```python
from build123d import *

# Parameters (mm, degrees)
BOSS_EXTRU_1_DEPTH      = 6
CONG_1_R                = 3
CONG_2_R                = 20
ENL_V_MAT_EXTRU_1_REACH = 118.402
ESQUISSE2_R             = 1.45
ENL_V_MAT_EXTRU_2_REACH = 118.402
CONG_3_R                = 1.5
ESQUISSE4_R             = 1.45
ENL_V_MAT_EXTRU_3_DEPTH = 6
ESQUISSE5_R             = 1.15
ENL_V_MAT_EXTRU_4_DEPTH = 6


with BuildPart() as part:
    # Esquisse1 → Boss.-Extru.1 (new body)
    with BuildSketch(Plane.XY):
        with BuildLine():
            Line((-14, -30), (-5.970001079, -110))
            ThreePointArc((-5.970001079, -110), (0, -115.400761222), (5.970001079, -110))
            Line((5.970001079, -110), (14, -30))
            Line((14, -30), (14, -18))
            Line((14, -18), (-6, -18))
            Line((-6, -18), (-6, 22))
            Line((-6, 22), (14, 22))
            Line((14, 22), (14, 30))
            Line((14, 30), (-14, 30))
            Line((-14, 30), (-14, -30))
        make_face()
    extrude(amount=BOSS_EXTRU_1_DEPTH)

    # Congé1
    cong_1_edges = [part.edges().sort_by_distance(p)[0] for p in [
        (-14, 30, 3),
        (14, 30, 3),
    ]]
    fillet(cong_1_edges, radius=CONG_1_R)

    # Congé2
    cong_2_edges = [part.edges().sort_by_distance(p)[0] for p in [
        (14, -30, 3),
        (-14, -30, 3),
    ]]
    fillet(cong_2_edges, radius=CONG_2_R)

    # Esquisse2 → Enlèv. mat.-Extru.1 (cut, up to next)
    with BuildSketch(Plane.XY.offset(6), mode=Mode.PRIVATE) as enl_v_mat_extru_1_sk1:
        with Locations((9.08, -21.75)):
            Circle(ESQUISSE2_R)
    enl_v_mat_extru_1_tool1 = extrude(enl_v_mat_extru_1_sk1.sketch, amount=-ENL_V_MAT_EXTRU_1_REACH, mode=Mode.PRIVATE) & part.part
    # Esquisse2 → Enlèv. mat.-Extru.1 (cut, up to next)
    with BuildSketch(Plane.XY.offset(6), mode=Mode.PRIVATE) as enl_v_mat_extru_1_sk2:
        with Locations((-1.08, -21.75)):
            Circle(ESQUISSE2_R)
    enl_v_mat_extru_1_tool2 = extrude(enl_v_mat_extru_1_sk2.sketch, amount=-ENL_V_MAT_EXTRU_1_REACH, mode=Mode.PRIVATE) & part.part
    # Esquisse2 → Enlèv. mat.-Extru.1 (cut, up to next)
    with BuildSketch(Plane.XY.offset(6), mode=Mode.PRIVATE) as enl_v_mat_extru_1_sk3:
        with Locations((-1.08, 25.75)):
            Circle(ESQUISSE2_R)
    enl_v_mat_extru_1_tool3 = extrude(enl_v_mat_extru_1_sk3.sketch, amount=-ENL_V_MAT_EXTRU_1_REACH, mode=Mode.PRIVATE) & part.part
    # Esquisse2 → Enlèv. mat.-Extru.1 (cut, up to next)
    with BuildSketch(Plane.XY.offset(6), mode=Mode.PRIVATE) as enl_v_mat_extru_1_sk4:
        with Locations((9.08, 25.75)):
            Circle(ESQUISSE2_R)
    enl_v_mat_extru_1_tool4 = extrude(enl_v_mat_extru_1_sk4.sketch, amount=-ENL_V_MAT_EXTRU_1_REACH, mode=Mode.PRIVATE) & part.part
    add(enl_v_mat_extru_1_tool1.solids().sort_by_distance((9.08, -21.75, 6))[0], mode=Mode.SUBTRACT)
    add(enl_v_mat_extru_1_tool2.solids().sort_by_distance((-1.08, -21.75, 6))[0], mode=Mode.SUBTRACT)
    add(enl_v_mat_extru_1_tool3.solids().sort_by_distance((-1.08, 25.75, 6))[0], mode=Mode.SUBTRACT)
    add(enl_v_mat_extru_1_tool4.solids().sort_by_distance((9.08, 25.75, 6))[0], mode=Mode.SUBTRACT)

    # Esquisse3 → Enlèv. mat.-Extru.2 (cut, up to next)
    with BuildSketch(Plane.XY.offset(6), mode=Mode.PRIVATE) as enl_v_mat_extru_2_sk1:
        Polygon((-7.886583597, -31.017533633), (-4.584381628, -63.916187805), (6.894740823, -42.63737417), align=None)
    enl_v_mat_extru_2_tool1 = extrude(enl_v_mat_extru_2_sk1.sketch, amount=-ENL_V_MAT_EXTRU_2_REACH, mode=Mode.PRIVATE) & part.part
    # Esquisse3 → Enlèv. mat.-Extru.2 (cut, up to next)
    with BuildSketch(Plane.XY.offset(6), mode=Mode.PRIVATE) as enl_v_mat_extru_2_sk2:
        Polygon((6.894740823, -52.121802831), (-3.854189345, -70.511493223), (3.66385974, -84.30991259), align=None)
    enl_v_mat_extru_2_tool2 = extrude(enl_v_mat_extru_2_sk2.sketch, amount=-ENL_V_MAT_EXTRU_2_REACH, mode=Mode.PRIVATE) & part.part
    # Esquisse3 → Enlèv. mat.-Extru.2 (cut, up to next)
    with BuildSketch(Plane.XY.offset(6), mode=Mode.PRIVATE) as enl_v_mat_extru_2_sk3:
        Polygon((-2.728137467, -80.682315655), (-0.663223344, -101.254314661), (3.006387716, -91.078168987), align=None)
    enl_v_mat_extru_2_tool3 = extrude(enl_v_mat_extru_2_sk3.sketch, amount=-ENL_V_MAT_EXTRU_2_REACH, mode=Mode.PRIVATE) & part.part
    add(enl_v_mat_extru_2_tool1.solids().sort_by_distance((-1.858741, -45.857032, 6))[0], mode=Mode.SUBTRACT)
    add(enl_v_mat_extru_2_tool2.solids().sort_by_distance((2.234804, -68.98107, 6))[0], mode=Mode.SUBTRACT)
    add(enl_v_mat_extru_2_tool3.solids().sort_by_distance((-0.128324, -91.004933, 6))[0], mode=Mode.SUBTRACT)

    # Congé3
    cong_3_edges = [part.edges().sort_by_distance(p)[0] for p in [
        (6.894740823, -52.121802831, 3),
        (3.66385974, -84.30991259, 3),
        (-3.854189345, -70.511493223, 3),
        (-2.728137467, -80.682315655, 3),
        (3.006387716, -91.078168987, 3),
        (-0.663223344, -101.254314661, 3),
        (-7.886583597, -31.017533633, 3),
        (6.894740823, -42.63737417, 3),
        (-4.584381628, -63.916187805, 3),
    ]]
    fillet(cong_3_edges, radius=CONG_3_R)

    # Esquisse4 → Enlèv. mat.-Extru.3 (cut)
    with BuildSketch(Plane.XY.offset(6)):
        with Locations((0, -104.400761222)):
            Circle(ESQUISSE4_R)
    extrude(amount=-ENL_V_MAT_EXTRU_3_DEPTH, mode=Mode.SUBTRACT)

    # Esquisse5 → Enlèv. mat.-Extru.4 (cut)
    with BuildSketch(Plane.XY.offset(6)):
        with Locations((-8.41, 17)):
            Circle(ESQUISSE5_R)
        with Locations((-8.41, 7)):
            Circle(ESQUISSE5_R)
    extrude(amount=-ENL_V_MAT_EXTRU_4_DEPTH, mode=Mode.SUBTRACT)


solid = part.part
```
Input: part model. Units: mm. Frame: model coordinates. A direction names the side the tool comes from. Coordinates: 2 decimals unless noted, no trailing zeros. Loops run counter-clockwise (first coordinate to the right, second up) from the corner with the lowest first, then second, coordinate; pieces in that order, holes last. Notation, with made-up numbers: M 17,15 L 67,15 A17 ccw 67,46 Z; hole C 71.25,76.5 d7. An arc over 180 degrees is marked long. Use a Markdown table: item, result. Add a question column.
1) Set-up query: faces 5 (the cylindrical face through (-13.1, 29.14, 3.04)), 6 (the flat face through (4, 22, 3)), 7 (the flat face through (0.044, -63.842, 3.042)). Return all of +Z, -Z, +X, -X, +Y, -Y with unobstructed straight access to the full face (end or side cutting, diameter ignored); none if empty.
2) Section D-D, the plane z = 1.25. Give the number of separate pieces and of enclosed holes in the cut face, plus the area to 3 significant figures.
3) Section B-B, the plane x = 9.08. Return the cut outline in (y, z).
4) Section C-C, the plane y = -63. Return the cut outline in (x, z).
5) Line query: L1, parallel to Y at x = 0.75, z = 1.75; L2, parallel to X at y = 18, z = 4.25; L3, parallel to X at y = -73.5, z = 5. Output: solid intervals per line, ascending. Write a range as from..to.
6) Draft query along X for faces 1 (the cylindrical face through (-0.1, -115.4, 3)), 2 (the cylindrical face through (5.21, -57.41, 2.96)), 3 (the cylindrical face through (10.419, -22.305, 3.042)), 4 (the flat face through (6, -41.7, 6)). Return one class per face: +X half, -X half, draft (parallel to the pull), parting line (faces both ways), or undercut.
7) Section A-A, the plane y = 25.75. Return the cut outline in (x, z), plus the area to 3 significant figures.
8) Pin query (flat end, axial travel): P1, Ø1.4, axis at x = -8.41, y = 7, coming from the +Z side; P2, Ø1.8, axis at y = 3, z = 2, coming from the +X side; P3, Ø1, axis at x = 5, z = 5, coming from the -Y side; P4, Ø1.8, axis at x = 5.5, z = 2.5, coming from the -Y side. Return the tip coordinate at first contact, or that it passes through.
Answer below:
| question | item | result |
|---|---|---|
| 1 | face 5 | +Z, -Z, -X, +Y |
| 1 | face 6 | +Z, -Z, +X |
| 1 | face 7 | +Z, -Z |
| 2 | separate pieces | 1 |
| 2 | enclosed holes | 10 |
| 2 | area | 2,100 mm2 |
| 3 | outline | M -79.02,0 L -23.2,0 L -23.2,6 L -79.02,6 Z; M -20.3,0 L -18,0 L -18,6 L -20.3,6 Z; M 22,0 L 24.3,0 L 24.3,6 L 22,6 Z; M 27.2,0 L 30,0 L 30,6 L 27.2,6 Z |
| 4 | outline | M -10.69,0 L 0.54,0 L 0.54,6 L -10.69,6 Z; M 5.8,0 L 10.69,0 L 10.69,6 L 5.8,6 Z |
| 5 | L1 | -115.35..-105.64, -103.16..-95.91, -87..-78.96, -62.63..-54.03, -37.81..-18, 22..30 |
| 5 | L2 | -14..-8.98, -7.84..-6 |
| 5 | L3 | -9.63..-2.23, 4.75..9.63 |
| 6 | face 1 | parting line |
| 6 | face 2 | undercut |
| 6 | face 3 | undercut |
| 6 | face 4 | draft |
| 7 | outline | M -14,0 L -2.53,0 L -2.53,6 L -14,6 Z; M 0.37,0 L 7.63,0 L 7.63,6 L 0.37,6 Z; M 10.53,0 L 14,0 L 14,6 L 10.53,6 Z |
| 7 | area | 133 mm2 |
| 8 | P1 | through |
| 8 | P2 | x = -6 |
| 8 | P3 | y = -113.37 |
| 8 | P4 | y = -113.25 |
